Source: CAD feature listing. Evaluate the final solid. Frame: model axes, mm. Round coordinates to 2 decimals unless told otherwise and drop trailing zeros. Order: outer loops, then holes, each group sorted by start corner. A loop starts at its lowest first (then second) coordinate and runs counter-clockwise, first axis right, second up. Notation, with made-up numbers: (67, 60.25) -> (114, 60.25) arc R4 ccw to (114, 66.25) -> close; hole circle Ø8 at (-36.75, 46). An arc over 180 degrees is marked (long way). Answer as CSV lines item,"result". Start each with the question number.
(1) Contact query for flat-ended pins moving along their axis: P1, Ø1.5, axis at x = 191.5, y = 238.5, coming from the +Z side; P2, Ø6, axis at y = 315.5, z = -290.5, coming from the -X side; P3, Ø4, axis at x = 203.5, y = 244.5, coming from the -Z side. Output: stop coordinate, or through.
(2) Section query C-C (z = -159.5). Output: boundary loops of the cut face in (x, y).
(3) Section query D-D (y = 123). Output: boundary loops of the cut face in (x, z), plus the area to 3 significant figures.
(4) Section query B-B (y = 269). Output: boundary loops of the cut face in (x, z), plus the area to 3 significant figures.
(5) Line query: line 1 along Y through (x, z) = (275, -185); line 2 along X through (y, z) = (240, -67.5); line 3 along Z through (x, y) = (265, 327). Output: solid intervals per line, ascending. Write a range as from..to.
(6) Section query A-A (x = 129.5). Output: boundary loops of the cut face in (y, z).
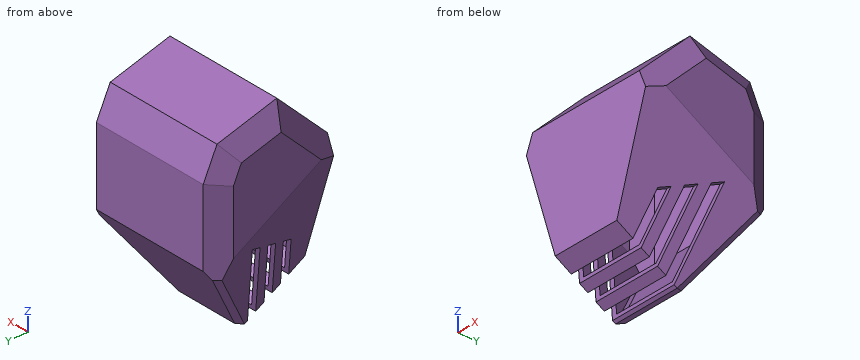
```python
from build123d import *
from OCP.BRepFilletAPI import BRepFilletAPI_MakeChamfer

# Parameters (mm, degrees)
BOSS_EXTRU_1_DEPTH      = 310
CHANFREIN1_SIZE         = 80
CHANFREIN1_SIZE2        = 219.798193556
CHANFREIN2_SIZE         = 25
CHANFREIN2_SIZE2        = 43.301270189
CHANFREIN3_SIZE         = 10
CHANFREIN3_SIZE2        = 11.000628676
CHANFREIN3_SIZE2_2      = 10.311972297
COQUE1_T                = 10
ENL_V_MAT_EXTRU_1_DEPTH = 657.524942405


with BuildPart() as part:
    # Esquisse1 → Boss.-Extru.1 (new body)
    with BuildSketch(Plane(origin=(0, 0, 0), x_dir=(0, 0, -1), z_dir=(1, 0, 0))):
        Polygon((369.170962313, 100), (450, 240), (264.340759124, 370), (99.168602631, 370), (34.833395016, 340), (0, 210), (110, 100), align=None)
    extrude(amount=BOSS_EXTRU_1_DEPTH)

    # Chanfrein1
    chanfrein1_edges = [part.edges().sort_by_distance(p)[0] for p in [
        (310, 170, -409.585481157),
        (0, 170, -409.585481157),
    ]]
    chanfrein1_side = [part.faces().sort_by_distance(p)[0] for p in [
        (155, 170, -409.585481157),
    ]]
    chamfer(chanfrein1_edges, length=CHANFREIN1_SIZE, length2=CHANFREIN1_SIZE2, reference=chanfrein1_side[0])

    # Chanfrein2: one chamfer whose edges measure the first distance from different faces: ONE call of the kernel's chamfer builder (chamfer() names one face for all edges)
    chanfrein2_edges_1 = [part.edges().sort_by_distance(p)[0] for p in [
        (0, 155, -55),
        (310, 155, -55),
    ]]
    chanfrein2_side_1 = [part.faces().sort_by_distance(p)[0] for p in [
        (155, 155, -55),
    ]]
    chanfrein2_edges_2 = [part.edges().sort_by_distance(p)[0] for p in [
        (0, 275, -17.416697508),
        (310, 275, -17.416697508),
    ]]
    chanfrein2_side_2 = [part.faces().sort_by_distance(p)[0] for p in [
        (155, 275, -17.416697508),
    ]]
    chanfrein2_edges_3 = [part.edges().sort_by_distance(p)[0] for p in [
        (0, 355, -67.000998824),
        (310, 355, -67.000998824),
    ]]
    chanfrein2_side_3 = [part.faces().sort_by_distance(p)[0] for p in [
        (155, 355, -67.000998824),
    ]]
    chanfrein2_edges_4 = [part.edges().sort_by_distance(p)[0] for p in [
        (0, 370, -181.754680877),
        (310, 370, -181.754680877),
    ]]
    chanfrein2_side_4 = [part.faces().sort_by_distance(p)[0] for p in [
        (155, 370, -181.754680877),
    ]]
    chanfrein2 = BRepFilletAPI_MakeChamfer(part.part.solid().wrapped)
    for e in chanfrein2_edges_1:
        chanfrein2.Add(CHANFREIN2_SIZE, CHANFREIN2_SIZE2, e.wrapped, chanfrein2_side_1[0].wrapped)  # the first distance lies on this face
    for e in chanfrein2_edges_2:
        chanfrein2.Add(CHANFREIN2_SIZE, CHANFREIN2_SIZE2, e.wrapped, chanfrein2_side_2[0].wrapped)  # the first distance lies on this face
    for e in chanfrein2_edges_3:
        chanfrein2.Add(CHANFREIN2_SIZE, CHANFREIN2_SIZE2, e.wrapped, chanfrein2_side_3[0].wrapped)  # the first distance lies on this face
    for e in chanfrein2_edges_4:
        chanfrein2.Add(CHANFREIN2_SIZE, CHANFREIN2_SIZE2, e.wrapped, chanfrein2_side_4[0].wrapped)  # the first distance lies on this face
    add(Compound.cast(chanfrein2.Shape()), mode=Mode.REPLACE)

    # Chanfrein3: one chamfer whose edges measure the first distance from different faces: ONE call of the kernel's chamfer builder (chamfer() names one face for all edges)
    chanfrein3_edges_1 = [part.edges().sort_by_distance(p)[0] for p in [
        (155, 240, -450),
    ]]
    chanfrein3_side_1 = [part.faces().sort_by_distance(p)[0] for p in [
        (155, 170, -409.585481157),
    ]]
    chanfrein3_edges_2 = [part.edges().sort_by_distance(p)[0] for p in [
        (46.013035878, 293.764248554, -373.216695593),
    ]]
    chanfrein3_side_2 = [part.faces().sort_by_distance(p)[0] for p in [
        (36.692430522, 203.807514508, -291.710403206),
    ]]
    chanfrein3_edges_3 = [part.edges().sort_by_distance(p)[0] for p in [
        (263.986964122, 293.764248554, -373.216695593),
    ]]
    chanfrein3_side_3 = [part.faces().sort_by_distance(p)[0] for p in [
        (273.307569478, 203.807514508, -291.710403206),
    ]]
    chanfrein3 = BRepFilletAPI_MakeChamfer(part.part.solid().wrapped)
    for e in chanfrein3_edges_1:
        chanfrein3.Add(CHANFREIN3_SIZE, CHANFREIN3_SIZE2, e.wrapped, chanfrein3_side_1[0].wrapped)  # the first distance lies on this face
    for e in chanfrein3_edges_2:
        chanfrein3.Add(CHANFREIN3_SIZE, CHANFREIN3_SIZE2_2, e.wrapped, chanfrein3_side_2[0].wrapped)  # the first distance lies on this face
    for e in chanfrein3_edges_3:
        chanfrein3.Add(CHANFREIN3_SIZE, CHANFREIN3_SIZE2_2, e.wrapped, chanfrein3_side_3[0].wrapped)  # the first distance lies on this face
    add(Compound.cast(chanfrein3.Shape()), mode=Mode.REPLACE)

    # Coque1 (no face opened: a closed hollow body)
    add(offset(amount=-COQUE1_T, mode=Mode.PRIVATE), mode=Mode.SUBTRACT)

    # Esquisse2 → Enlèv. mat.-Extru.1 (cut, through all)
    with BuildSketch(Plane(origin=(0, 0, 0), x_dir=(0, 0, -1), z_dir=(1, 0, 0))):
        Polygon((441.142030756, 224.657547217), (256.142030756, 274.228147817), (264.492620752, 251.285090363), (430.789268951, 206.726037773), align=None)
        Polygon((297.894980737, 159.512860546), (389.378221735, 135), (399.730983539, 152.931509443), (289.544390741, 182.455918), align=None)
        Polygon((272.843210748, 228.342032908), (281.193800745, 205.398975454), (410.083745343, 170.863018887), (420.436507147, 188.79452833), align=None)
    extrude(amount=ENL_V_MAT_EXTRU_1_DEPTH, mode=Mode.SUBTRACT)


solid = part.part
```
Answer block:
1,P1,"z = -7.44"
1,P2,"x = 14.89"
1,P3,"z = -442.01"
2,outline,"(0, 176.44) -> (13.91, 100) -> (296.09, 100) -> (310, 176.44) -> (310, 326.7) -> (285, 370) -> (25, 370) -> (0, 326.7) -> close; hole (10, 179.96) -> (22.73, 110) -> (287.27, 110) -> (300, 179.96) -> (300, 324.02) -> (279.23, 360) -> (30.77, 360) -> (10, 324.02) -> close"
3,outline,"(3.48, -139.7) -> (80, -382.45) -> (230, -382.45) -> (306.52, -139.7) -> (285, -87) -> (25, -87) -> close; hole (14.52, -140.95) -> (87, -370.9) -> (223, -370.9) -> (295.48, -140.95) -> (279.23, -101.14) -> (30.77, -101.14) -> close"
3,area,"11,300 mm2"
4,outline,"(0, -212.94) -> (14.22, -258.04) -> (24.86, -258.04) -> (10, -210.91) -> (10, -63.41) -> (30.77, -26.16) -> (279.23, -26.16) -> (300, -63.41) -> (300, -210.91) -> (285.14, -258.04) -> (295.78, -258.04) -> (310, -212.94) -> (310, -60.64) -> (285, -15.81) -> (25, -15.81) -> (0, -60.64) -> close; (19.77, -275.65) -> (56.17, -391.16) -> (72.64, -408.58) -> (237.36, -408.58) -> (253.83, -391.16) -> (290.23, -275.65) -> (279.59, -275.65) -> (245.62, -383.42) -> (238.32, -391.15) -> (71.68, -391.15) -> (64.38, -383.42) -> (30.41, -275.65) -> close"
4,area,"13,200 mm2"
5,line 1,"100..110, 360..370"
5,line 2,"0..10, 300..310"
5,line 3,"-325.75..-308.32, -41.7..-31.35"
6,outline,"(100, -369.17) -> (135, -389.38) -> (137.68, -379.38) -> (110, -363.4) -> (110, -114.14) -> (212.99, -11.15) -> (332.91, -43.29) -> (360, -101.39) -> (360, -261.19) -> (240.21, -432.27) -> (232.75, -434.27) -> (227.34, -431.14) -> (224.66, -441.14) -> (231.34, -445) -> (246.31, -440.99) -> (370, -264.34) -> (370, -99.17) -> (340, -34.83) -> (210, 0) -> (100, -110) -> close; (152.93, -399.73) -> (170.86, -410.08) -> (173.54, -400.08) -> (155.61, -389.73) -> close; (188.79, -420.44) -> (206.73, -430.79) -> (209.41, -420.79) -> (191.47, -410.44) -> close"
